CAD build for the part. Positions are in the model's coordinates, mm. A direction names the side the tool comes from. Give positions to 0.01 mm unless a question says otherwise; leave off trailing zeros. Loops run counter-clockwise (first coordinate to the right, second up) from the corner with the lowest first, then second, coordinate; pieces in that order, holes last.
```python
from build123d import *

# Parameters (mm, degrees)
SKETCH1_R            = 72.5
SKETCH1_R_2          = 4
BOSS_EXTRUDE1_DEPTH  = 35
CUT_EXTRUDE1_DEPTH   = 35
CIRPATTERN6_COUNT    = 3
MIRROR2_COPY_1_DEPTH = 35
MIRROR2_COPY_2_DEPTH = 35


with BuildPart() as part:
    # Sketch1 → Boss-Extrude1 (new body)
    with BuildSketch(Plane.XY):
        Circle(SKETCH1_R)
        Circle(SKETCH1_R_2, mode=Mode.SUBTRACT)
    extrude(amount=BOSS_EXTRUDE1_DEPTH)

    # Sketch3 → Cut-Extrude1 (cut)
    with BuildSketch(Plane.XY.offset(35)):
        with BuildLine():
            Line((0, 38.272172541), (0, 8.722907964))
            ThreePointArc((0, 8.722907964), (-3.329803479, 8.062352767), (-6.155298303, 6.180730228))
            Line((-6.155298303, 6.180730228), (-16.518963046, 34.523659292))
            ThreePointArc((-16.518963046, 34.523659292), (-8.469467098, 37.323281181), (0, 38.272172541))
        make_face()
    cut_extrude1 = extrude(amount=-CUT_EXTRUDE1_DEPTH, mode=Mode.SUBTRACT)

    # Mirror1: Cut-Extrude1 across plane
    add(cut_extrude1.mirror(Plane(origin=(0, 38.272172541, 0), x_dir=(0, 0, 1), z_dir=(1, 0, 0))), mode=Mode.SUBTRACT)

    # CirPattern6: Cut-Extrude1 ×3 about axis
    cirpattern6_axis = Axis((0, 0, 0), (0, 0, 1))
    for i in range(1, CIRPATTERN6_COUNT):
        add(cut_extrude1.rotate(cirpattern6_axis, i * 360 / CIRPATTERN6_COUNT), mode=Mode.SUBTRACT)

    # Mirror2: Cut-Extrude1 across plane
    add(cut_extrude1.mirror(Plane(origin=(33.144673679, -19.136086271, 0), x_dir=(0, 0, 1), z_dir=(-0.5000000000000041, -0.8660254037844364, 0))), mode=Mode.SUBTRACT)

    # Mirror2 copy 1 sketch → Mirror2 copy 1 (cut)
    with BuildSketch(Plane(origin=(0, 0, 35), x_dir=(-1, 0, 0), z_dir=(0, 0, 1))):
        with BuildLine():
            Line((0, -38.272172541), (0, -8.722907964))
            ThreePointArc((0, -8.722907964), (-3.329803479, -8.062352767), (-6.155298303, -6.180730228))
            Line((-6.155298303, -6.180730228), (-16.518963046, -34.523659292))
            ThreePointArc((-16.518963046, -34.523659292), (-8.469467098, -37.323281181), (0, -38.272172541))
        make_face()
    extrude(amount=-MIRROR2_COPY_1_DEPTH, mode=Mode.SUBTRACT)

    # Mirror2 copy 2 sketch → Mirror2 copy 2 (cut)
    with BuildSketch(Plane(origin=(0, 0, 35), x_dir=(0.5000000000000079, 0.8660254037844346, 0), z_dir=(0, 0, 1))):
        with BuildLine():
            Line((0, -38.272172541), (0, -8.722907964))
            ThreePointArc((0, -8.722907964), (-3.329803479, -8.062352767), (-6.155298303, -6.180730228))
            Line((-6.155298303, -6.180730228), (-16.518963046, -34.523659292))
            ThreePointArc((-16.518963046, -34.523659292), (-8.469467098, -37.323281181), (0, -38.272172541))
        make_face()
    extrude(amount=-MIRROR2_COPY_2_DEPTH, mode=Mode.SUBTRACT)


solid = part.part
```
1. Tool access for faces 4 (the face through (11.265, 20.154, 17.745)), 5 (the face through (-1, -15, 0)): list every direction of +Z, -Z, +X, -X, +Y, -Y with a clear straight run to the whole face (end or side of a thin tool).
Responses:
face 4: +Z, -Z
face 5: -Z, +X, -X, +Y, -Y
2. Saw through at C-C, the plane y = 0. List the corners of the cut face in (x, z), and give its area (3 significant figures).
Responses:
outline: (-72.5, 0) - (-21.25, 0) - (-21.25, 35) - (-72.5, 35) - close; (-8.72, 0) - (-4, 0) - (-4, 35) - (-8.72, 35) - close; (4, 0) - (8.72, 0) - (8.72, 35) - (4, 35) - close; (21.25, 0) - (72.5, 0) - (72.5, 35) - (21.25, 35) - close
area: 3,920 mm2
3. Saw through at B-B, the plane x = -26.5. List the corners of the cut face in (y, z).
Responses:
outline: (-67.48, 0) - (-27.61, 0) - (-27.61, 35) - (-67.48, 35) - close; (-0.92, 0) - (67.48, 0) - (67.48, 35) - (-0.92, 35) - close
4. Probe line 1 along Y through (x, z) = (0.5, 23.5); line 2 along X through (y, z) = (-16.5, 18); line 3 along X through (y, z) = (17, 25.5). List the from-to ranges inside material, lowest first.
Responses:
line 1: y = -72.5 to -3.97, 3.97 to 8.71, 38.27 to 72.5
line 2: x = -70.6 to -34.53, -9.03 to 9.03, 34.53 to 70.6
line 3: x = -70.48 to -10.11, 10.11 to 70.48
5. Saw through at A-A, the plane z = 10.5. List the corners of the cut face in (x, y).
Responses:
outline: circle Ø145 at (0, 0); hole (-38.16, -2.96) arc R38.27 ccw to (-21.64, -31.57) - (-2.28, -8.42) arc R8.72 cw to (-8.43, 2.24) - close; hole (-16.52, 34.52) - (-6.16, 6.18) arc R8.72 cw to (6.16, 6.18) - (16.52, 34.52) arc R38.27 ccw to start; hole circle Ø8 at (0, 0); hole (2.28, -8.42) - (21.64, -31.57) arc R38.27 ccw to (38.16, -2.96) - (8.43, 2.24) arc R8.72 cw to start
6. Pull direction Y, two halves, no side cores. Call faces 1 (the face through (-11.82, -19.83, 17.74)), 2 (the face through (69.15, 21.78, 17.26)), 3 (the face through (-1, -15, 35)): released by +Y, released by -Y, zero draft, split by the parting line, or undercut.
Responses:
face 1: undercut
face 2: split by the parting line
face 3: zero draft
7. Drop flat-ended pins along their axis: pin 1 (1.5 mm diameter, centred on x = 41.5, z = 30, fed in from +Y); pin 2 (10.5 mm diameter, centred on x = 0, y = 0, fed in from -Z); pin 3 (12 mm diameter, centred on x = -9.5, z = 26.5, fed in from +Y); pin 4 (1 mm diameter, centred on y = -16, z = 16.5, fed in from -X). Give the stop position or say it passes through.
Responses:
pin 1: stops at y = 59.96
pin 2: stops at z = 0
pin 3: stops at y = 72.42
pin 4: stops at x = -70.82
8. Saw through at D-D, the plane y = -17. List the corners of the cut face in (x, z), and give its area (3 significant figures).
Responses:
outline: (-70.48, 0) - (-34.29, 0) - (-34.29, 35) - (-70.48, 35) - close; (-9.45, 0) - (9.45, 0) - (9.45, 35) - (-9.45, 35) - close; (34.29, 0) - (70.48, 0) - (70.48, 35) - (34.29, 35) - close
area: 3,190 mm2
